Geometry: see drawing. Coordinates: mm, zero at the bounding-box minimum. A direction names the side the tool comes from. Round coordinates to 2 decimals unless told otherwise and drop trailing zeros. Order: outer loops, then holes, each group sorted by start corner. A loop starts at its lowest first (then second) coordinate and runs counter-clockwise, first axis right, second up. Notation, with made-up numbers: (75.5, 88) -> (93.5, 88) arc R28 ccw to (93.5, 121) -> close; hole circle Ø10 at (33.25, 31.25). An arc over 180 degrees is marked (long way). Put each result on its own line as item: value.
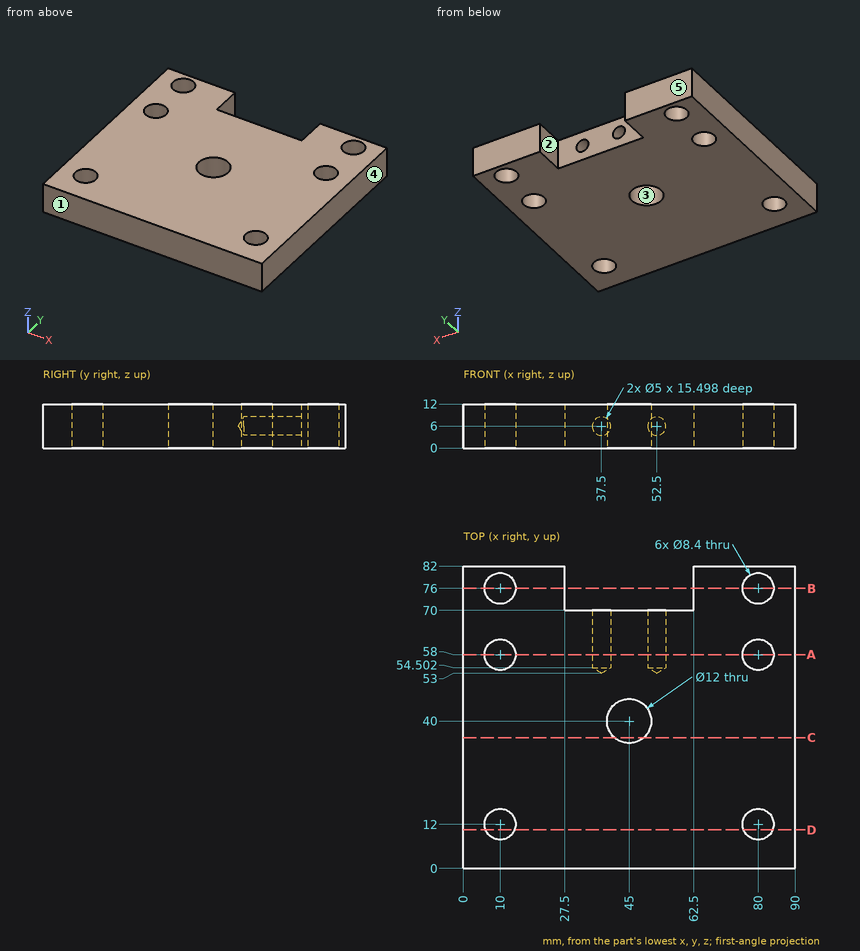
1. Cut plane D-D on y = 10.5. Return loops of the section in (x, z).
Ans:
outline: (0, 0) -> (6.08, 0) -> (6.08, 12) -> (0, 12) -> close; (13.92, 0) -> (76.08, 0) -> (76.08, 12) -> (13.92, 12) -> close; (83.92, 0) -> (90, 0) -> (90, 12) -> (83.92, 12) -> close
2. Material intervals for probe 1 along Y at (x, z) = (80, 2.75); probe 2 along Y at (x, z) = (13, 1.5); probe 3 along X at (y, z) = (15, 2.5), sorted ascending.
Ans:
probe 1: 0 to 7.8, 16.2 to 53.8, 62.2 to 71.8, 80.2 to 82
probe 2: 0 to 9.06, 14.94 to 55.06, 60.94 to 73.06, 78.94 to 82
probe 3: 0 to 7.06, 12.94 to 77.06, 82.94 to 90
3. Draft query along Y for the marked faces 3, 4 and 5. Return one class per face: +Y half, -Y half, draft (parallel to the pull), parting line (faces both ways), or undercut.
Ans:
face 3: undercut
face 4: draft
face 5: +Y half
4. Contact query for flat-ended pins moving along their axis: P1, Ø4.5, axis at x = 52.5, z = 6, coming from the +Y side; P2, Ø7, axis at x = 45, y = 40, coming from the +Z side; P3, Ø3, axis at x = 37.5, z = 6, coming from the +Y side. Output: stop coordinate, or through.
Ans:
P1: y = 54.35
P2: through
P3: y = 53.9
5. Cut plane C-C on y = 35.5. Return loops of the section in (x, z), and give its area (3 significant figures).
Ans:
outline: (0, 0) -> (41.03, 0) -> (41.03, 12) -> (0, 12) -> close; (48.97, 0) -> (90, 0) -> (90, 12) -> (48.97, 12) -> close
area: 985 mm²
6. Cut plane A-A on y = 58. Return loops of the section in (x, z).
Ans:
outline: (0, 0) -> (5.8, 0) -> (5.8, 12) -> (0, 12) -> close; (14.2, 0) -> (75.8, 0) -> (75.8, 12) -> (14.2, 12) -> close; (84.2, 0) -> (90, 0) -> (90, 12) -> (84.2, 12) -> close; hole circle Ø5 at (37.5, 6); hole circle Ø5 at (52.5, 6)
7. Set-up query: the marked faces 1 and 2. Return all of +Z, -Z, +X, -X, +Y, -Y with unobstructed straight access to the full face (end or side cutting, diameter ignored); none if empty.
Ans:
face 1: +Z, -Z, +X, -X, -Y
face 2: +Z, -Z, +Y
8. Cut plane B-B on y = 76. Return loops of the section in (x, z).
Ans:
outline: (0, 0) -> (5.8, 0) -> (5.8, 12) -> (0, 12) -> close; (14.2, 0) -> (27.5, 0) -> (27.5, 12) -> (14.2, 12) -> close; (62.5, 0) -> (75.8, 0) -> (75.8, 12) -> (62.5, 12) -> close; (84.2, 0) -> (90, 0) -> (90, 12) -> (84.2, 12) -> close
